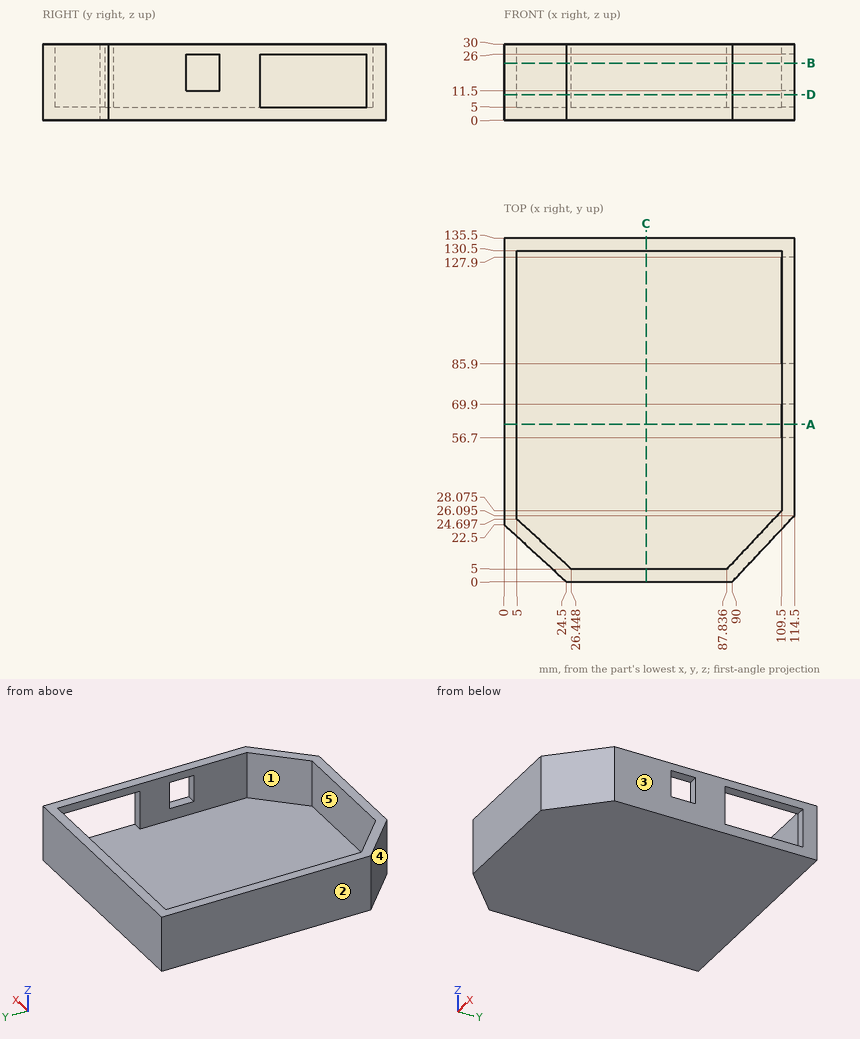
Check sheet for the drawn part. Datum: minimum x, y, z corner. Units: mm. A direction names the side the tool comes from. Coordinates: 2 decimals unless noted, no trailing zeros. Order: outer loops, then holes, each group sorted by start corner. A loop starts at its lowest first (then second) coordinate and runs counter-clockwise, first axis right, second up. Notation, with made-up numbers: M 29,34.25 L 42,34.25 A21 cw 42,66.25 Z; hole C -36,57.5 d1. An arc over 180 degrees is marked long. One line per question, with ' | ' between items. Start each with the question number.
Item 1: Material ranges on line 1 (Y direction, x = 84, z = 11); line 2 (X direction, y = 87, z = 28); line 3 (X direction, y = 117.5, z = 6), recorded low to high.
Item 2: Gauge pin test, flat ends, axial feed: P1, Ø5.5, axis at x = 113, z = 20.5, coming from the -Y side; P2, Ø5, axis at x = 36, y = 93, coming from the +Z side; P3, Ø1.5, axis at x = 112.5, z = 16.5, coming from the -Y side (1 decimal). Record the tip position at first contact, or that the pin passes through.
Item 3: Access from +Z, -Z, +X, -X, +Y, -Y to the whole of each face (thin tool, end or side, straight path). Record for the marked faces 1 and 2.
Item 4: Sectioned sample at A-A on y = 62. Record the cut outline in (x, z), and give its area (3 significant figures).
Item 5: Mould release check, pull along Y, two halves, no side actions. Record for the marked faces 3, 4 and 5: pulls with the +Y half, pulls with the -Y half, needs draft (parallel to the pull), parting line crosses it, or undercut.
Item 6: Sectioned sample at C-C on x = 56. Record the cut outline in (y, z).
Item 7: Sectioned sample at B-B on z = 22.5. Record the cut outline in (x, y) (1 decimal).
Item 8: Sectioned sample at D-D on z = 10. Record the cut outline in (x, y) (1 decimal).
Answer below:
1) line 1: y = 0 to 5, 130.5 to 135.5 | line 2: x = 0 to 5, 109.5 to 114.5 | line 3: x = 0 to 5
2) P1: stops at y = 21.57 | P2: stops at z = 5 | P3: stops at y = 23.2
3) face 1: +Z | face 2: +Z, -Z, -X, +Y, -Y
4) outline: M 0,0 L 114.5,0 L 114.5,11.5 L 109.5,11.5 L 109.5,5 L 5,5 L 5,30 L 0,30 Z; M 109.5,26 L 114.5,26 L 114.5,30 L 109.5,30 Z | area: 750 mm^2
5) face 3: needs draft | face 4: pulls with the -Y half | face 5: undercut
6) outline: M 0,0 L 135.5,0 L 135.5,30 L 130.5,30 L 130.5,5 L 5,5 L 5,30 L 0,30 Z
7) outline: M 0,22.5 L 24.5,0 L 90,0 L 114.5,26.1 L 114.5,56.7 L 109.5,56.7 L 109.5,28.1 L 87.8,5 L 26.4,5 L 5,24.7 L 5,130.5 L 109.5,130.5 L 109.5,127.9 L 114.5,127.9 L 114.5,135.5 L 0,135.5 Z; M 109.5,69.9 L 114.5,69.9 L 114.5,85.9 L 109.5,85.9 Z
8) outline: M 0,22.5 L 24.5,0 L 90,0 L 114.5,26.1 L 114.5,85.9 L 109.5,85.9 L 109.5,28.1 L 87.8,5 L 26.4,5 L 5,24.7 L 5,130.5 L 109.5,130.5 L 109.5,127.9 L 114.5,127.9 L 114.5,135.5 L 0,135.5 Z
